Part model, mm, in its own coordinate system. Face numbers are marked on the shaded views. A direction names the side the tool comes from. Round coordinates to 2 decimals unless told otherwise and drop trailing zeros. Order: outer loops, then holes, each group sorted by start corner. A loop starts at its lowest first (then second) coordinate and runs counter-clockwise, first axis right, second up. Notation, with made-up numbers: (89, 79) - (129, 79) arc R9 ccw to (129, 85) - close; hole circle Ø5 at (-27, 22). An arc over 180 degrees is marked (long way). Answer as a JSON object with one key per item and string values.
Autodesk Inventor part; units mm, degrees
ref_plane "YZ Plane" through (0, 0, 0) normal (1, 0, 0) x (0, 1, 0)
ref_plane "XZ Plane" through (0, 0, 0) normal (0, 1, 0) x (-1, 0, 0)
ref_plane "XY Plane" through (0, 0, 0) normal (0, 0, 1) x (1, 0, 0)
sketch "Sketch1" plane through (0, 0, 0) normal (0, 1, 0) x (-1, 0, 0)
  line L0 (49.6871, 42.6052) -> (39.6871, 32.6052)
  line L1 (53.8292, 42.6052) -> (49.6871, 42.6052)
  line L2 (53.8292, 27.6052) -> (53.8292, 42.6052)
  line L3 (68.8292, 27.6052) -> (53.8292, 27.6052)
  line L4 (68.8292, 23.4631) -> (68.8292, 27.6052)
  line L5 (58.8292, 13.4631) -> (68.8292, 23.4631)
  line L6 (53.8292, 13.4631) -> (58.8292, 13.4631)
  line L7 (39.6871, 27.6052) -> (53.8292, 13.4631)
  line L8 (39.6871, 32.6052) -> (39.6871, 27.6052)
  line L9 (58.8292, 13.4631) -> (53.8292, 13.4631)
  line L10 (58.8292, 13.4631) -> (16.4028, -28.9633)
  line L11 (16.4028, -28.9633) -> (11.4028, -28.9633)
  line L12 (11.4028, -28.9633) -> (-2.7393, -14.8212)
  line L13 (-2.7393, -14.8212) -> (-2.7393, -9.8212)
  line L14 (-2.7393, -9.8212) -> (39.6871, 32.6052)
  line L15 (39.6871, 27.6052) -> (39.6871, 32.6052)
  line L16 (53.8292, 13.4631) -> (39.6871, 27.6052)
  circle A0 centre (13.9028, -12.3212) radius 11.15
  line L17 (53.8292, 27.6052) -> (53.8292, -37.3948)
  line L18 (53.8292, 27.6052) -> (-11.1708, 27.6052)
  line L19 (53.8292, -37.3948) -> (49.8292, -37.3948)
  line L20 (49.8292, -37.3948) -> (49.8292, -12.3948)
  line L21 (49.8292, -12.3948) -> (32.9714, -12.3948)
  line L22 (-11.1708, 27.6052) -> (-11.1708, 23.6052)
  line L23 (-11.1708, 23.6052) -> (13.8292, 23.6052)
  line L24 (13.8292, 23.6052) -> (13.8292, 6.7473)
  point P0 (0, 0)
  dimension "d5" = 65
  dimension "d6" = 4
  dimension "d7" = 25
extrude "Extrusion1" add sketch "Sketch1" against normal blind 15 contours L18 L17 L7 | L7 L17 L10 L11 L12 L13 L14 L18 | L14 L24 L23 L22 L18 | L17 L19 L20 L21 L10
sketch "Sketch2" plane through (0, -15, 0) normal (0, -1, 0) x (1, 0, 0)
  circle A0 centre (-13.9028, -12.3212) radius 11.15
  circle A1 centre (-13.9028, -12.3212) radius 7.5
  point P0 (0, 0)
  dimension "d2" = 15
extrude "Extrusion2" add sketch "Sketch2" against normal blind 9
sketch "Sketch3" plane through (0, 0, 0) normal (0, 1, 0) x (1, 0, 0)
  line L0 (2.7393, 14.8212) -> (-11.4028, 28.9633)
  line L1 (-11.4028, 28.9633) -> (-16.4028, 28.9633)
  line L2 (-16.4028, 28.9633) -> (-32.9714, 12.3948)
  line L3 (-32.9714, 12.3948) -> (-49.8292, 12.3948)
  line L4 (-49.8292, 12.3948) -> (-49.8292, 37.3948)
  line L5 (-49.8292, 37.3948) -> (-53.8292, 37.3948)
  line L6 (-53.8292, 37.3948) -> (-53.8292, -27.6052)
  line L7 (-53.8292, -27.6052) -> (11.1708, -27.6052)
  line L8 (11.1708, -27.6052) -> (11.1708, -23.6052)
  line L9 (11.1708, -23.6052) -> (-13.8292, -23.6052)
  line L10 (-13.8292, -23.6052) -> (-13.8292, -6.7473)
  line L11 (-13.8292, -6.7473) -> (2.7393, 9.8212)
  line L12 (2.7393, 9.8212) -> (2.7393, 14.8212)
  circle A0 centre (-13.9028, 12.3212) radius 11.15
  line L13 (2.7393, 14.8212) -> (11.1708, 6.3898)
  line L14 (11.1708, 6.3898) -> (11.1708, -23.6052)
  line L15 (-11.4028, 28.9633) -> (-19.8343, 37.3948)
  line L16 (-19.8343, 37.3948) -> (-49.8292, 37.3948)
  line L17 (-11.4028, 28.9633) -> (-16.4028, 28.9633)
  point P0 (0, 0)
extrude "Extrusion3" add sketch "Sketch3" against normal blind 2 contours L13 L14 L9 L10 L11 L12 | L1 L2 L3 L4 L16 L15
sketch "Sketch4" plane through (0, -15, 0) normal (0, -1, 0) x (1, 0, 0)
  line L0 (2.7393, -9.8212) -> (-13.8292, 6.7473)
  line L1 (2.7393, -14.8212) -> (2.7393, -9.8212)
  line L2 (2.7393, -14.8212) -> (11.1708, -6.3898)
  line L3 (11.1708, -6.3898) -> (11.1708, 23.6052)
  line L4 (-13.8292, 23.6052) -> (11.1708, 23.6052)
  line L5 (-13.8292, 6.7473) -> (-13.8292, 23.6052)
  line L6 (-49.8292, -37.3948) -> (-19.8343, -37.3948)
  line L7 (-19.8343, -37.3948) -> (-11.4028, -28.9633)
  line L8 (-16.4028, -28.9633) -> (-11.4028, -28.9633)
  line L9 (-32.9714, -12.3948) -> (-16.4028, -28.9633)
  line L10 (-49.8292, -12.3948) -> (-32.9714, -12.3948)
  line L11 (-49.8292, -37.3948) -> (-49.8292, -12.3948)
  point P0 (0, 0)
extrude "Extrusion4" add sketch "Sketch4" against normal blind 2
sketch "Sketch5" plane through (11.1708, -2, 23.6052) normal (0, 0, -1) x (-1, 0, 0)
  line L0 (0, -11) -> (25, -11)
  line L1 (25, 0) -> (25, -11)
  line L2 (25, 0) -> (0, 0)
  line L3 (0, 0) -> (0, -11)
  point P0 (11.1708, 2)
  point P1 (12.5, -5.5)
  point P2 (0, -5.5)
  point P3 (12.5, 0)
hole "Hole1" at (-1.3292, -7.5, 23.6052) direction (0, 0, 1) diameter 3.5 end through all
sketch "Sketch6" plane through (-49.8292, -2, -12.3948) normal (1, 0, 0) x (0, 0, -1)
  line L0 (0, -11) -> (25, -11)
  line L1 (25, 0) -> (25, -11)
  line L2 (25, 0) -> (0, 0)
  line L3 (0, 0) -> (0, -11)
  point P0 (-12.3948, 2)
  point P1 (12.5, -5.5)
  point P2 (25, -5.5)
  point P3 (12.5, 0)
hole "Hole2" at (-49.8292, -7.5, -24.8948) direction (-1, 0, 0) diameter 3.5 end through all
sketch "Sketch7" plane through (0, 0, 0) normal (0, 1, 0) x (1, 0, 0)
  line L0 (11.1708, 6.3898) -> (-19.8343, 37.3948)
  line L1 (-19.8343, 37.3948) -> (-53.8292, 37.3948)
  line L2 (-53.8292, 37.3948) -> (-53.8292, -27.6052)
  line L3 (-53.8292, -27.6052) -> (11.1708, -27.6052)
  line L4 (11.1708, -27.6052) -> (11.1708, 6.3898)
  circle A0 centre (-13.9028, 12.3212) radius 11.15
  line L5 (-48.8292, -22.6052) -> (-48.8292, 7.3948)
  circle A1 centre (-13.9028, 12.3212) radius 16.15
  line L6 (-48.8292, -22.6052) -> (-18.8292, -22.6052)
  line L7 (-18.8292, -22.6052) -> (-18.8292, -3.0591)
  line L8 (-48.8292, 7.3948) -> (-29.2831, 7.3948)
  point P0 (0, 0)
  dimension "d26" = 5
  dimension "d27" = 5
  dimension "d28" = 5
  dimension "d31" = 30
extrude "Extrusion5" cut sketch "Sketch7" against normal through all contours A1 L7 L6 L5 L8
equation "\"d27\" = d28"
properties part number "Z Axis Bottom Bearing Holder" material "ABS Plastic"
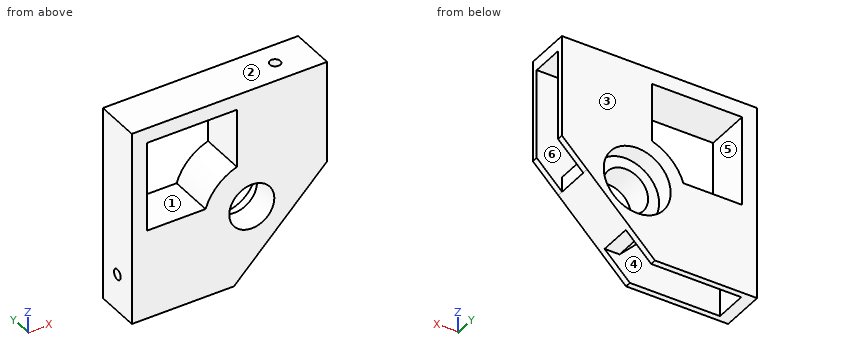
Item 1: Tool access for the marked faces 1 and 2: list every direction of +Z, -Z, +X, -X, +Y, -Y with a clear straight run to the whole face (end or side of a thin tool).
Taken from the geometry:
{"face 1": "+Y, -Y", "face 2": "+Z, +X, -X, +Y, -Y"}
Item 2: Cut at B-B (y = -7.5). Write the cut outline in (x, z), plus the area to 3 significant figures.
Taken from the geometry:
{"outline": "(-53.83, -37.39) - (-49.83, -37.39) - (-49.83, -26.64) - (-53.83, -26.64) - close; (-53.83, -23.14) - (-49.83, -23.14) - (-49.83, -12.39) - (-32.97, -12.39) - (-16.4, -28.96) - (-11.4, -28.96) - (2.74, -14.82) - (2.74, -9.82) - (-13.83, 6.75) - (-13.83, 23.61) - (-3.08, 23.61) - (-3.08, 27.61) - (-53.83, 27.61) - close; (0.42, 23.61) - (11.17, 23.61) - (11.17, 27.61) - (0.42, 27.61) - close; hole (-48.83, -7.39) - (-29.28, -7.39) arc R16.15 cw to (-18.83, 3.06) - (-18.83, 22.61) - (-48.83, 22.61) - close; hole circle Ø15 at (-13.9, -12.32)", "area": "1,300 mm2"}
Item 3: Drop flat-ended pins along their axis: P1, Ø1.5, axis at x = -14, y = -8, coming from the -Z side; P2, Ø2, axis at x = -46.5, y = -3.5, coming from the -Z side; P3, Ø9, axis at x = 4.5, y = -7.5, coming from the -Z side. Give the stop position or say it passes through.
Taken from the geometry:
{"P1": "z = -28.96", "P2": "z = -12.39", "P3": "z = -17.56"}
Item 4: Cut at A-A (z = 21). Write the cut outline in (x, y), plus the area to 3 significant figures.
Taken from the geometry:
{"outline": "(-53.83, -15) - (-48.83, -15) - (-48.83, 0) - (-53.83, 0) - close; (-18.83, -15) - (11.17, -15) - (11.17, -13) - (-13.83, -13) - (-13.83, -2) - (11.17, -2) - (11.17, 0) - (-18.83, 0) - close", "area": "250 mm2"}
Item 5: Cut at D-D (x = 4). Write the cut outline in (y, z), plus the area to 3 significant figures.
Taken from the geometry:
{"outline": "(-15, -13.56) - (-13, -13.56) - (-13, 23.61) - (-2, 23.61) - (-2, -13.56) - (0, -13.56) - (0, 27.61) - (-15, 27.61) - close", "area": "209 mm2"}
Item 6: Cut at C-C (x = -44.5). Write the cut outline in (y, z).
Taken from the geometry:
{"outline": "(-15, -37.39) - (-13, -37.39) - (-13, -12.39) - (-2, -12.39) - (-2, -37.39) - (0, -37.39) - (0, -7.39) - (-15, -7.39) - close; (-15, 22.61) - (0, 22.61) - (0, 27.61) - (-15, 27.61) - close"}
Item 7: Probe L1, parallel to X at y = -1, z = 22.5; L2, parallel to X at y = -9, z = 15.5; L3, parallel to Z at x = -9, y = -3.25. List the from-to ranges inside material, lowest first. Write a range as from..to.
Taken from the geometry:
{"L1": "-53.83..-48.83, -18.83..11.17", "L2": "-53.83..-48.83, -18.83..-13.83", "L3": "-26.56..-22.34, -2.31..1.92, 23.61..27.61"}
Item 8: Two-plate mould, pull along Y, no slides. Class the marked faces 3, 4, 5 and 6: pulls with the +Y half, pulls with the -Y half, needs draft (parallel to the pull), parting line crosses it, or undercut.
Taken from the geometry:
{"face 3": "pulls with the +Y half", "face 4": "undercut", "face 5": "needs draft", "face 6": "undercut"}
